Model file for the job. Use its own axes, mm. Coordinates: 2 decimals unless noted, no trailing zeros. Order: outer loops, then holes, each group sorted by start corner. A loop starts at its lowest first (then second) coordinate and runs counter-clockwise, first axis right, second up. Notation, with made-up numbers: (-2.75, 64.25) -> (7.25, 64.25) arc R10 ccw to (7.25, 69.25) -> close; hole circle Ø3 at (-6, -31). An arc over 180 degrees is marked (long way). Return JSON: item names as keys, results as strings. Group by question number.
1) Cut at B-B (y = 0). Write the cut outline in (x, z) (3 decimals).
2) Flat gauge pin, fed straight in: pin 1 (5 mm diameter, centred on x = 9, y = 4.5, fed in from -Z). Where does the tip first touch, or does it go through?
3) Probe line 1 (Y direction, x = 19.5, z = 0.5) (3 decimals); line 2 (X direction, y = -0.25, z = 0.9); line 3 (Y direction, x = -18.5, z = 0.85). List the from-to ranges inside material, lowest first.
4) Cut at A-A (x = -19.5). Write the cut outline in (y, z) (3 decimals).
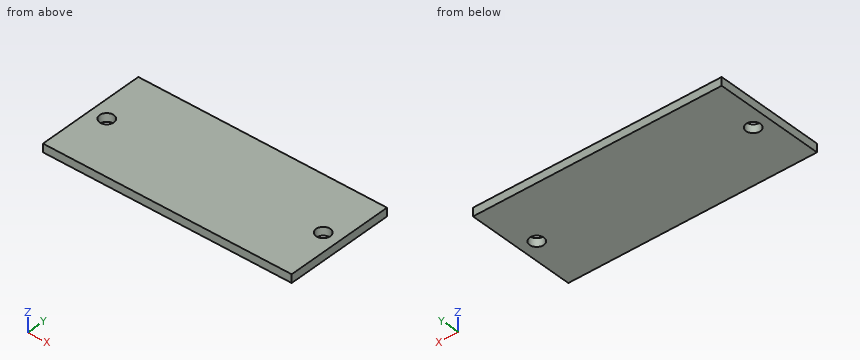
from build123d import *

# Parameters (mm, degrees)
SKETCH2_W           = 44.8
SKETCH2_H           = 19.8
BOSS_EXTRUDE1_DEPTH = 1.5
SKETCH3_R           = 1.275
CUT_EXTRUDE1_DEPTH  = 25.536095859


with BuildPart() as part:
    # Sketch2 → Boss-Extrude1 (new body)
    with BuildSketch(Plane.XY):
        Rectangle(SKETCH2_W, SKETCH2_H)
    extrude(amount=BOSS_EXTRUDE1_DEPTH)

    # Sketch3 → Cut-Extrude1 (cut, through all)
    with BuildSketch(Plane.XY.offset(1.5)):
        with Locations((-19.5, 0)):
            Circle(SKETCH3_R)
    cut_extrude1 = extrude(amount=-CUT_EXTRUDE1_DEPTH, mode=Mode.SUBTRACT)

    # Mirror1: Cut-Extrude1 across plane
    add(cut_extrude1.mirror(Plane(origin=(0, 0, 0), x_dir=(0, 0, 1), z_dir=(1, 0, 0))), mode=Mode.SUBTRACT)


solid = part.part
Answers below:
{
 "1": {"outline": "(-22.4, 0) -> (-20.775, 0) -> (-20.775, 1.5) -> (-22.4, 1.5) -> close; (-18.225, 0) -> (18.225, 0) -> (18.225, 1.5) -> (-18.225, 1.5) -> close; (20.775, 0) -> (22.4, 0) -> (22.4, 1.5) -> (20.775, 1.5) -> close"},
 "2": {"pin 1": "stops at z = 0"},
 "3": {"line 1": "y = -9.9 to -1.275, 1.275 to 9.9", "line 2": "x = -22.4 to -20.75, -18.25 to 18.25, 20.75 to 22.4", "line 3": "y = -9.9 to -0.79, 0.79 to 9.9"},
 "4": {"outline": "(-9.9, 0) -> (-1.275, 0) -> (-1.275, 1.5) -> (-9.9, 1.5) -> close; (1.275, 0) -> (9.9, 0) -> (9.9, 1.5) -> (1.275, 1.5) -> close"}
}
